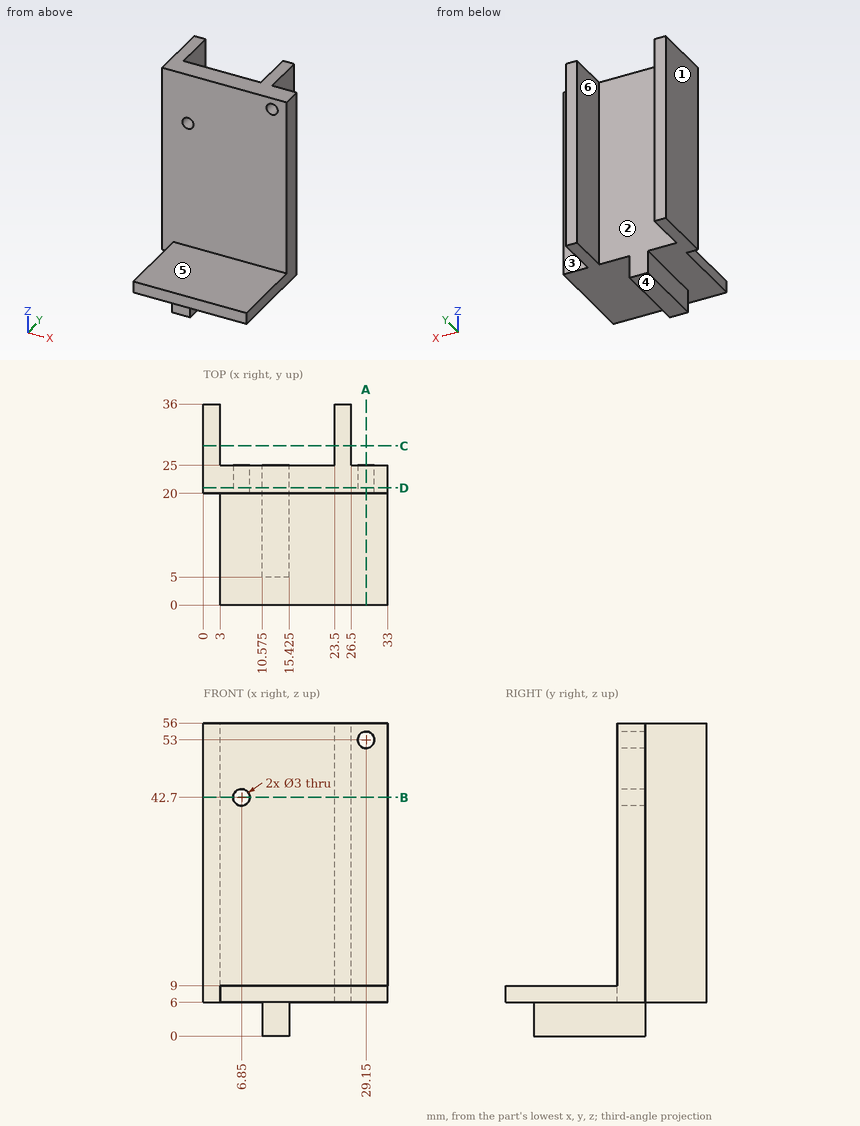
Drawing for the job (mm, zero at the part's lowest x, y, z). A direction names the side the tool comes from. Coordinates: 2 decimals unless noted, no trailing zeros. Write each loop counter-clockwise with the first axis right and the second up, starting at its lowest first coordinate (ties: lowest second). Pieces come first, ordered by that corner, then holes. Notation, with made-up numbers: (-30, 55.5) - (-9, 55.5) arc R13 cw to (-9, 59.5) - close; hole circle Ø9 at (13.25, -3.75). An arc over 180 degrees is marked (long way). Write each question's results on one line, items separated by ' | '. Start each with the question number.
1) Mould opens along X. For the marked faces 1, 2 and 3 say: pulls with the +X half, pulls with the -X half, needs draft (parallel to the pull), parting line crosses it, or undercut.
2) Cut at C-C (y = 28.5). Write the cut outline in (x, z).
3) Probe line 1 along Z through (x, y) = (29.15, 21.5); line 2 along X through (y, z) = (33.5, 30); line 3 along X through (y, z) = (21.25, 42.7). List the from-to ranges inside material, lowest first. Write a range as from..to.
4) Cut at A-A (x = 29.15). Write the cut outline in (y, z), then the cut area to 3 significant figures.
5) 3-axis set-ups, long thin cutter, end or side, ignore diameter. For the marked faces 4, 5 and 6: which of +Z, -Z, +X, -X, +Y, -Y reach the whole face in a straight line?
6) Flat gauge pins, fed straight in: P1, Ø3, axis at x = 21, z = 36, coming from the -Y side; P2, Ø0.9, axis at y = 9.5, z = 7, coming from the -X side; P3, Ø4, axis at x = 6.85, z = 42.7, coming from the +Y side. Where does each tip first touch, or does it go through?
7) Cut at D-D (y = 21). Write the cut outline in (x, z) (3 decimals).
8) Cut at B-B (z = 42.7). Write the cut outline in (x, y).
Returned:
1) face 1: pulls with the -X half | face 2: undercut | face 3: needs draft
2) outline: (0, 6) - (3, 6) - (3, 56) - (0, 56) - close; (23.5, 6) - (26.5, 6) - (26.5, 56) - (23.5, 56) - close
3) line 1: 6..51.5, 54.5..56 | line 2: 0..3, 23.5..26.5 | line 3: 0..5.35, 8.35..33
4) outline: (0, 6) - (25, 6) - (25, 51.5) - (20, 51.5) - (20, 9) - (0, 9) - close; (20, 54.5) - (25, 54.5) - (25, 56) - (20, 56) - close | area: 295 mm^2
5) face 4: -Z, +X, -X, +Y, -Y | face 5: +Z, +X, -X, -Y | face 6: +Z, -Z, +Y
6) P1: y = 20 | P2: x = 3 | P3: y = 25
7) outline: (0, 6) - (10.575, 6) - (10.575, 0) - (15.425, 0) - (15.425, 6) - (33, 6) - (33, 56) - (0, 56) - close; hole circle Ø3 at (6.85, 42.7); hole circle Ø3 at (29.15, 53)
8) outline: (0, 20) - (5.35, 20) - (5.35, 25) - (3, 25) - (3, 36) - (0, 36) - close; (8.35, 20) - (33, 20) - (33, 25) - (26.5, 25) - (26.5, 36) - (23.5, 36) - (23.5, 25) - (8.35, 25) - close
